```python
from build123d import *

# Parameters (mm, degrees)
SKETCH1_W            = 157.864
SKETCH1_H            = 90.551
BOSS_EXTRUDE1_DEPTH  = 8
CUT_EXTRUDE21_DEPTH  = 5
FILLET8_R            = 2.75
SKETCH29_W           = 12.37533
SKETCH29_H           = 90.551
CUT_EXTRUDE25_DEPTH  = 183.166204596
FILLET9_R            = 5
SKETCH36_W           = 10
SKETCH36_H           = 10
SKETCH36_R           = 3.3
BOSS_EXTRUDE10_DEPTH = 8
FILLET10_R           = 2.5
SKETCH37_R           = 7.5
CUT_EXTRUDE26_DEPTH  = 3


with BuildPart() as part:
    # Sketch1 → Boss-Extrude1 (new body)
    with BuildSketch(Plane(origin=(0, 0, 0), x_dir=(1, 0, 0), z_dir=(0, 1, 0))):
        with Locations((78.932, -45.2755)):
            Rectangle(SKETCH1_W, SKETCH1_H)
    extrude(amount=BOSS_EXTRUDE1_DEPTH)

    # Sketch23 → Cut-Extrude21 (cut)
    with BuildSketch(Plane(origin=(0, 8, 0), x_dir=(1, 0, 0), z_dir=(0, 1, 0))):
        Polygon((141.332, -86.4755), (23.3181173, -86.4755), (16.532, -79.6893827), (16.532, -10.8616173), (23.3181173, -4.0755), (141.332, -4.0755), align=None)
    extrude(amount=-CUT_EXTRUDE21_DEPTH, mode=Mode.SUBTRACT)

    # Fillet8
    fillet8_edges = [part.edges().sort_by_distance(p)[0] for p in [
        (141.332, 5.5, 4.0755),
        (141.332, 5.5, 86.4755),
        (23.3181173, 5.5, 86.4755),
        (16.532, 5.5, 79.6893827),
        (16.532, 5.5, 10.8616173),
        (23.3181173, 5.5, 4.0755),
    ]]
    fillet(fillet8_edges, radius=FILLET8_R)

    # Sketch29 → Cut-Extrude25 (cut, through all)
    with BuildSketch(Plane(origin=(0, 8, 0), x_dir=(1, 0, 0), z_dir=(0, 1, 0))):
        with Locations((151.676335, -45.2755)):
            Rectangle(SKETCH29_W, SKETCH29_H)
        with Locations((6.187665, -45.2755)):
            Rectangle(SKETCH29_W, SKETCH29_H)
    extrude(amount=-CUT_EXTRUDE25_DEPTH, mode=Mode.SUBTRACT)

    # Fillet9
    fillet9_edges = [part.edges().sort_by_distance(p)[0] for p in [
        (145.48867, 4, 90.551),
        (145.48867, 4, 0),
        (12.37533, 4, 0),
        (12.37533, 4, 90.551),
    ]]
    fillet(fillet9_edges, radius=FILLET9_R)

    # Sketch36 → Boss-Extrude10 (add)
    # profile 1 of 4: a face of its own
    with BuildSketch(Plane.XZ):
        with Locations((26.3936, 95.551)):
            Rectangle(SKETCH36_W, SKETCH36_H)
        with Locations(Location((26.3936, 95.551, 0), (0, 0, 270))):
            Circle(SKETCH36_R, mode=Mode.SUBTRACT)
    # profile 2 of 4: a face of its own
    with BuildSketch(Plane.XZ):
        with Locations((129.6936, 95.551)):
            Rectangle(SKETCH36_W, SKETCH36_H)
        with Locations(Location((129.6936, 95.551, 0), (0, 0, 270))):
            Circle(SKETCH36_R, mode=Mode.SUBTRACT)
    # profile 3 of 4: a face of its own
    with BuildSketch(Plane.XZ):
        with Locations((26.3936, -5)):
            Rectangle(SKETCH36_W, SKETCH36_H)
        with Locations(Location((26.3936, -5, 0), (0, 0, 270))):
            Circle(SKETCH36_R, mode=Mode.SUBTRACT)
    # profile 4 of 4: a face of its own
    with BuildSketch(Plane.XZ):
        with Locations((129.6936, -5)):
            Rectangle(SKETCH36_W, SKETCH36_H)
        with Locations(Location((129.6936, -5, 0), (0, 0, 270))):
            Circle(SKETCH36_R, mode=Mode.SUBTRACT)
    extrude(amount=-BOSS_EXTRUDE10_DEPTH)

    # Fillet10
    fillet10_edges = [part.edges().sort_by_distance(p)[0] for p in [
        (21.3936, 4, 90.551),
        (21.3936, 4, 100.551),
        (31.3936, 4, 100.551),
        (31.3936, 4, 90.551),
        (124.6936, 4, 90.551),
        (124.6936, 4, 100.551),
        (134.6936, 4, 100.551),
        (134.6936, 4, 90.551),
        (31.3936, 4, 0),
        (31.3936, 4, -10),
        (21.3936, 4, -10),
        (21.3936, 4, 0),
        (124.6936, 4, -10),
        (124.6936, 4, 0),
        (134.6936, 4, 0),
        (134.6936, 4, -10),
    ]]
    fillet(fillet10_edges, radius=FILLET10_R)

    # Sketch37 → Cut-Extrude26 (cut)
    with BuildSketch(Plane(origin=(0, 3, 0), x_dir=(1, 0, 0), z_dir=(0, 1, 0))):
        with Locations(Location((124.157, -72.2755, 0), (0, 0, 270))):
            Circle(SKETCH37_R)
        with Locations(Location((106.067, -72.2755, 0), (0, 0, 270))):
            Circle(SKETCH37_R)
        with Locations(Location((87.977, -72.2755, 0), (0, 0, 270))):
            Circle(SKETCH37_R)
        with Locations(Location((69.887, -72.2755, 0), (0, 0, 270))):
            Circle(SKETCH37_R)
        with Locations(Location((51.797, -72.2755, 0), (0, 0, 270))):
            Circle(SKETCH37_R)
        with Locations(Location((33.707, -72.2755, 0), (0, 0, 270))):
            Circle(SKETCH37_R)
        with Locations(Location((106.067, -54.2755, 0), (0, 0, 270))):
            Circle(SKETCH37_R)
        with Locations(Location((87.977, -54.2755, 0), (0, 0, 270))):
            Circle(SKETCH37_R)
        with Locations(Location((69.887, -54.2755, 0), (0, 0, 270))):
            Circle(SKETCH37_R)
        with Locations(Location((51.797, -54.2755, 0), (0, 0, 270))):
            Circle(SKETCH37_R)
        with Locations(Location((33.707, -54.2755, 0), (0, 0, 270))):
            Circle(SKETCH37_R)
        with Locations(Location((106.067, -36.2755, 0), (0, 0, 270))):
            Circle(SKETCH37_R)
        with Locations(Location((87.977, -36.2755, 0), (0, 0, 270))):
            Circle(SKETCH37_R)
        with Locations(Location((69.887, -36.2755, 0), (0, 0, 270))):
            Circle(SKETCH37_R)
        with Locations(Location((51.797, -36.2755, 0), (0, 0, 270))):
            Circle(SKETCH37_R)
        with Locations(Location((33.707, -36.2755, 0), (0, 0, 270))):
            Circle(SKETCH37_R)
        with Locations(Location((106.067, -18.2755, 0), (0, 0, 270))):
            Circle(SKETCH37_R)
        with Locations(Location((87.977, -18.2755, 0), (0, 0, 270))):
            Circle(SKETCH37_R)
        with Locations(Location((69.887, -18.2755, 0), (0, 0, 270))):
            Circle(SKETCH37_R)
        with Locations(Location((51.797, -18.2755, 0), (0, 0, 270))):
            Circle(SKETCH37_R)
        with Locations(Location((33.707, -18.2755, 0), (0, 0, 270))):
            Circle(SKETCH37_R)
        with Locations(Location((124.157, -54.2755, 0), (0, 0, 270))):
            Circle(SKETCH37_R)
        with Locations(Location((124.157, -36.2755, 0), (0, 0, 270))):
            Circle(SKETCH37_R)
        with Locations(Location((124.157, -18.2755, 0), (0, 0, 270))):
            Circle(SKETCH37_R)
    extrude(amount=-CUT_EXTRUDE26_DEPTH, mode=Mode.SUBTRACT)


solid = part.part
```
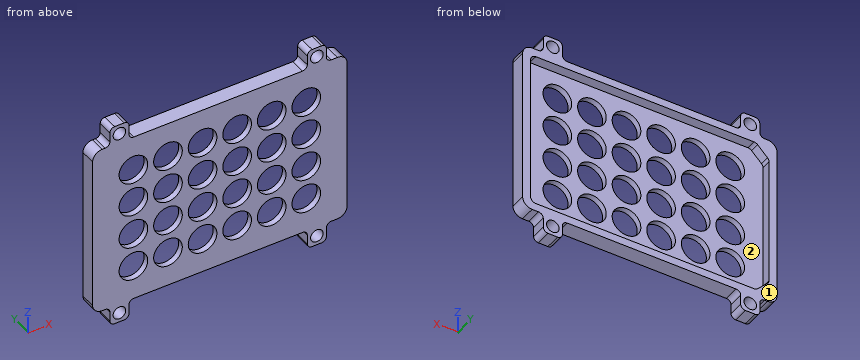
CAD build for the part. Positions are in the model's coordinates, mm. Face numbers are marked on the shaded views. Coordinates: 2 decimals unless noted, no trailing zeros. Write each loop counter-clockwise with the first axis right and the second up, starting at its lowest first coordinate (ties: lowest second). Pieces come first, ordered by that corner, then holes. Notation, with made-up numbers: (-0.5, -37.5) -> (3.5, -37.5) arc R22 cw to (3.5, -20.5) -> close; hole circle Ø2 at (4, -19). An arc over 180 degrees is marked (long way). Use CSV: the item, a comma, the result in double quotes. Start each with the question number.
Item 1: Band-saw the part on D-D, the plane x = 55. Write the cut outline in (y, z), plus the area to 3 significant figures.
Item 2: Band-saw the part on A-A, the plane z = -5. Write the cut outline in (x, y).
Item 3: Band-saw the part on C-C, the plane z = 15. Give the number of separate pieces and of enclosed holes in the cut face, plus the area to 3 significant figures.
Item 4: Wall check: probe 1 along Z at (x, y) = (73.5, 7.5); probe 2 along Z at (x, y) = (85, 2.75); probe 3 along X at (y, z) = (3.5, 33). Give the ranges that are in metal, low to high.
Item 5: Band-saw the part on B-B, the plane x = 75.5. Write the cut outline in (y, z), plus the area to 3 significant figures.
Item 6: Drop flat-ended pins along their axis: P1, Ø19.5, axis at x = 106.07, z = 36.28, coming from the -Y side; P2, Ø9, axis at x = 87.98, z = 36.28, coming from the -Y side; P3, Ø4, axis at y = 2, z = -5.5, coming from the +X side; P4, Ø2, axis at x = 92.5, y = 6, coming from the +Z side. Give the stop position or say it passes through.
Item 7: Two-plate mould, pull along Z, no slides. Class the marked faces 1 and 2: +Z half, -Z half, draft (parallel to the pull), parting line (faces both ways), or undercut.
Response values:
1,outline,"(0, 0) -> (8, 0) -> (8, 4.08) -> (3, 4.08) -> (3, 11.49) -> (0, 11.49) -> close; (0, 25.06) -> (3, 25.06) -> (3, 29.49) -> (0, 29.49) -> close; (0, 43.06) -> (3, 43.06) -> (3, 47.49) -> (0, 47.49) -> close; (0, 61.06) -> (3, 61.06) -> (3, 65.49) -> (0, 65.49) -> close; (0, 79.06) -> (3, 79.06) -> (3, 86.48) -> (8, 86.48) -> (8, 90.55) -> (0, 90.55) -> close"
1,area,"150 mm2"
2,outline,"(21.39, 0) -> (23.09, 0) -> (23.09, 8) -> (21.39, 8) -> close; (29.69, 0) -> (31.39, 0) -> (31.39, 8) -> (29.69, 8) -> close; (124.69, 0) -> (126.39, 0) -> (126.39, 8) -> (124.69, 8) -> close; (132.99, 0) -> (134.69, 0) -> (134.69, 8) -> (132.99, 8) -> close"
3,separate pieces,"7"
3,enclosed holes,"0"
3,area,"198 mm2"
4,probe 1,"z = 0 to 4.08, 86.48 to 90.55"
4,probe 2,"z = 0 to 11.39, 25.16 to 29.39, 43.16 to 47.39, 61.16 to 65.39, 79.16 to 90.55"
4,probe 3,"x = 12.38 to 16.53, 141.33 to 145.49"
5,outline,"(0, 0) -> (8, 0) -> (8, 4.08) -> (3, 4.08) -> (3, 13.3) -> (0, 13.3) -> close; (0, 23.25) -> (3, 23.25) -> (3, 31.3) -> (0, 31.3) -> close; (0, 41.25) -> (3, 41.25) -> (3, 49.3) -> (0, 49.3) -> close; (0, 59.25) -> (3, 59.25) -> (3, 67.3) -> (0, 67.3) -> close; (0, 77.25) -> (3, 77.25) -> (3, 86.48) -> (8, 86.48) -> (8, 90.55) -> (0, 90.55) -> close"
5,area,"193 mm2"
6,P1,"stops at y = 0"
6,P2,"passes through"
6,P3,"stops at x = 134.69"
6,P4,"stops at z = 90.55"
7,face 1,"draft"
7,face 2,"undercut"
